Read the model definition and answer for the solid it produces. Units are mm, in the model's axes. A direction names the side the tool comes from. Coordinates: 2 decimals unless noted, no trailing zeros. Loops run counter-clockwise (first coordinate to the right, second up) from the corner with the lowest first, then second, coordinate; pieces in that order, holes last. Notation, with made-up numbers: M -29,-32.5 L 18,-32.5 A16 cw 18,-15.5 Z; hole C 17,61 d11. An arc over 180 degrees is marked long. Put each result on its own line as item: value.
from build123d import *

# Parameters (mm, degrees)
F0_R     = 52
F1_DEPTH = 10
F2_R     = 4.99999


# Not quite as in the source:
# - a fillet or chamfer is up to 0.001 mm smaller than in the source, because OpenCascade refuses the exact size


with BuildPart() as f1:
    # F0 (on Front) → F1 (new body)
    with BuildSketch(Plane.XZ):
        with BuildLine():
            Line((5, -84.7722557505), (5, -54.7722557505))
            ThreePointArc((5, -54.7722557505), (0, 55), (-5, -54.7722557505))
            Line((-5, -54.7722557505), (-5, -84.7722557505))
            Line((-5, -84.7722557505), (5, -84.7722557505))
        make_face()
        Circle(F0_R, mode=Mode.SUBTRACT)
    extrude(amount=F1_DEPTH)

    # F2 (radius 5 in the source; OpenCascade refuses exactly that, so slightly less here)
    f2_edges = [f1.edges().sort_by_distance(p)[0] for p in [
        (5, -10, -69.772256),
        (-5, -10, -69.772256),
        (-5, 0, -69.772256),
        (5, 0, -69.772256),
    ]]
    fillet(f2_edges, radius=F2_R)


solid = f1.part
1) Given pin 1 Ø5 at (x, y) = (31.5, -4) entering from +Z; pin 2 Ø1 at (y, z) = (-1, 14.5) entering from +X; pin 3 Ø1.5 at (x, z) = (-6, -57.5) entering from -Y; pin 4 Ø1 at (x, y) = (-16.5, -2.5) entering from +Z, each flat-ended and moving along its own axis, determine where each tip first touches the part or whether it passes through.
Answer list:
pin 1: stops at z = 46.73
pin 2: stops at x = 53.19
pin 3: passes through
pin 4: stops at z = 52.62
2) Find section B-B, the plane x = 19.5. Write down the section's boundary in (y, z).
Answer list:
outline: M -10,-51.43 L 0,-51.43 L 0,-48.21 L -10,-48.21 Z; M -10,48.21 L 0,48.21 L 0,51.43 L -10,51.43 Z
3) Find section A-A, the plane z = 0. Write down the section's boundary in (x, y), plus the area to 3 significant figures.
Answer list:
outline: M -55,-10 L -52,-10 L -52,0 L -55,0 Z; M 52,-10 L 55,-10 L 55,0 L 52,0 Z
area: 60.0 mm^2
4) Straight lines are drawn through the part: line 1 (Z direction, x = -44.5, y = -1); line 2 (X direction, y = -0.5, z = 29); line 3 (Z direction, x = -30, y = -5.5). For each, find the intervals that lie inside material, in ascending order. Write a range as [from, to].
Answer list:
line 1: z = [-32.32, -26.9], [26.9, 32.32]
line 2: x = [-46.73, -43.16], [43.16, 46.73]
line 3: z = [-46.1, -42.47], [42.47, 46.1]
5) Determine the mould class of faces 1 (the cylindrical face through (2.418, -4.93, 54.947)), 2 (the flat face through (45, -10, 27)), 3 (the cylindrical face through (-41.265, -4.93, -31.641)), 4 (the flat face through (0, -5, -84.772)) for opening direction Z: released by +Z, released by -Z, zero draft, split by the parting line, or undercut.
Answer list:
face 1: split by the parting line
face 2: zero draft
face 3: undercut
face 4: released by -Z
6) Find section C-C, the plane y = -6.75. Write down the section's boundary in (x, z), plus the area to 3 significant figures.
Answer list:
outline: M -4.68,-84.77 L 4.68,-84.77 L 4.68,-54.8 A55 ccw long -4.68,-54.8 Z; hole C 0,0 d104
area: 1,290 mm^2
7) Which of the six approach directions +Z, -Z, +X, -X, +Y, -Y give full straight-line access (tool end or side, diameter ignored) to faces 5 (the cylindrical face through (4, -8, -70)), 6 (the cylindrical face through (4, -2, -70)), 7 (the cylindrical face through (-4, -2, -70)), 8 (the flat face through (45, 0, 27)), 9 (the cylindrical face through (-4, -8, -70))?
Answer list:
face 5: -Z, +X, -Y
face 6: -Z, +X, +Y
face 7: -Z, -X, +Y
face 8: +Z, -Z, +X, -X, +Y
face 9: -Z, -X, -Y
